Read the model definition and answer for the solid it produces. Units are mm, in the model's axes. A direction names the side the tool comes from. Coordinates: 2 decimals unless noted, no trailing zeros. Write each loop counter-clockwise with the first axis right and the second up, starting at its lowest first coordinate (ties: lowest second). Pieces come first, ordered by that corner, then holes.
Item 1: Section A-A (x = 28.5) is taken. Give the vertices of the cut face in (y, z).
Item 2: Section C-C (z = 0.4) is taken. Give the vertices of the cut face in (x, y), then the cut area to 3 significant figures.
Item 3: A tool of negligible diameter and unlimited length cuts with its end or side. For faces 5 (the face through (38.01, 19.51, 0.49)), 6 (the face through (31, 26.367, 1)), 7 (the face through (28, 16.367, 1)), from which of +Z, -Z, +X, -X, +Y, -Y can it reach the whole face along a straight path? Write none if from no direction.
Item 4: Section B-B (y = 18.25) is taken. Give the vertices of the cut face in (x, z), then the cut area to 3 significant figures.
Item 5: Section D-D (x = 35.75) is taken. Give the vertices of the cut face in (y, z), then the cut area to 3 significant figures.
Item 6: Straight lines are drawn through the part: probe 1 along Y at (x, z) = (35.96, 0.6); probe 2 along Y at (x, z) = (35.96, 2.3); probe 3 along X at (y, z) = (17, 0.4). For each, find the intervals that lie inside material, in ascending order.
Item 7: Determine the mould class of faces 1 (the face through (37, 18, 1)), 2 (the face through (33, 19, 0)), 3 (the face through (28, 21.367, 1)), 4 (the face through (43.46, 18.7, 1.48)) for opening direction Y: released by +Y, released by -Y, zero draft, split by the parting line, or undercut.
from build123d import *

# Parameters (mm, degrees)
MODEL_R                 = 1
SALIENTE_EXTRUIR1_DEPTH = 3
CROQUIS2_R              = 2.15
CORTAR_EXTRUIR1_DEPTH   = 1


with BuildPart() as part:
    # Model → Saliente-Extruir1 (new body)
    with BuildSketch(Plane.XY):
        with BuildLine():
            Line((26.66, 16.366878764), (26.66, 11.366878764))
            Line((26.66, 11.366878764), (35.96, 11.366878764))
            ThreePointArc((35.96, 11.366878764), (43.46, 18.866878764), (35.96, 26.366878764))
            Line((35.96, 26.366878764), (26.66, 26.366878764))
            Line((26.66, 26.366878764), (26.66, 21.366878764))
            Line((26.66, 21.366878764), (29.66, 21.366878764))
            Line((29.66, 21.366878764), (29.66, 16.366878764))
            Line((29.66, 16.366878764), (26.66, 16.366878764))
        make_face()
        with Locations((35.96, 18.866878764)):
            Circle(MODEL_R, mode=Mode.SUBTRACT)
    extrude(amount=SALIENTE_EXTRUIR1_DEPTH)

    # Croquis2 → Cortar-Extruir1 (cut)
    with BuildSketch(Plane.XY):
        with Locations((35.96, 18.866878764)):
            Circle(CROQUIS2_R)
    extrude(amount=CORTAR_EXTRUIR1_DEPTH, mode=Mode.SUBTRACT)


solid = part.part
Established:
1. outline: (11.37, 0) - (16.37, 0) - (16.37, 3) - (11.37, 3) - close; (21.37, 0) - (26.37, 0) - (26.37, 3) - (21.37, 3) - close
2. outline: (26.66, 11.37) - (35.96, 11.37) arc R7.5 ccw to (35.96, 26.37) - (26.66, 26.37) - (26.66, 21.37) - (29.66, 21.37) - (29.66, 16.37) - (26.66, 16.37) - close; hole circle Ø4.3 at (35.96, 18.87)
2. area: 198 mm2
3. face 5: -Z
3. face 6: +Z, -Z, +X, -X, +Y
3. face 7: +Z, -Z, -X
4. outline: (29.66, 0) - (33.9, 0) - (33.9, 1) - (35.17, 1) - (35.17, 3) - (29.66, 3) - close; (36.75, 1) - (38.02, 1) - (38.02, 0) - (43.43, 0) - (43.43, 3) - (36.75, 3) - close
4. area: 34.1 mm2
5. outline: (11.37, 0) - (16.73, 0) - (16.73, 1) - (17.89, 1) - (17.89, 3) - (11.37, 3) - close; (19.84, 1) - (21.01, 1) - (21.01, 0) - (26.37, 0) - (26.37, 3) - (19.84, 3) - close
5. area: 36.8 mm2
6. probe 1: y = 11.37 to 16.72, 21.02 to 26.37
6. probe 2: y = 11.37 to 17.87, 19.87 to 26.37
6. probe 3: x = 29.66 to 34.89, 37.03 to 43.22
7. face 1: undercut
7. face 2: zero draft
7. face 3: undercut
7. face 4: split by the parting line
